Autodesk Inventor part; units mm, degrees
ref_plane "YZ Plane" through (0, 0, 0) normal (1, 0, 0) x (0, 1, 0)
ref_plane "XZ Plane" through (0, 0, 0) normal (0, 1, 0) x (-1, 0, 0)
ref_plane "XY Plane" through (0, 0, 0) normal (0, 0, 1) x (1, 0, 0)
sketch "Esboço1" plane through (0, 0, 0) normal (0, 0, 1) x (1, 0, 0)
  circle A0 centre (0, 0) radius 4
  circle A1 centre (-7, 44.6) radius 3
  circle A2 centre (45, 0) radius 3
  circle A3 centre (-6, -44.6) radius 3
  circle A4 centre (-43.5, 11.3) radius 3
  circle A5 centre (0, 0) radius 29.3573
  circle A6 centre (-7, 44.6) radius 5
  circle A7 centre (-43.5, 11.3) radius 5
  circle A8 centre (-6, -44.6) radius 5
  circle A9 centre (45, 0) radius 5
  line L0 (-12, 44.6) -> (-12, 26.7927)
  line L1 (40.0933, -0.9613) -> (42.8631, -4.0842)
  line L2 (-2.5586, 46.8966) -> (6.9412, 28.5249)
  line L3 (-45.4208, 6.6836) -> (-29.3573, 0)
  line L4 (-42.4056, 16.1788) -> (-26.5097, 12.6129)
  line L5 (-9, -27.9437) -> (-10.963, -43.993)
  line L6 (1.5707, -29.3152) -> (-1.4137, -47.5322)
  line L7 (14.7039, 28.5249) -> (31.099, 28.5249)
  line L8 (31.099, 28.5249) -> (53.6238, -3.5874)
  line L9 (-48.496, 11.5007) -> (-48.496, 11.0993)
  line L10 (14.6238, -44.6) -> (14.6238, -108.4)
  line L11 (53.6238, -44.6) -> (53.6238, -108.4)
  line L12 (53.6238, -108.4) -> (14.6238, -108.4)
  line L13 (65.104, -44.6) -> (65.104, -19.9542)
  line L14 (65.104, -19.9542) -> (49.0934, 2.8713)
  line L15 (14.6238, -44.6) -> (14.6238, -25.4557)
  line L16 (-6, -44.6) -> (-0.9333, -44.6)
  line L17 (14.6238, -44.6) -> (65.104, -44.6)
  line L18 (14.7039, 28.5249) -> (6.9412, 28.5249)
  point P0 (-1, -44.6)
  dimension "d15" = 10
  dimension "d0" = 8
  dimension "d1" = 44.6
  dimension "d2" = 7
  dimension "d3" = 6
  dimension "d4" = 6
  dimension "d5" = 45
  dimension "d6" = 6
  dimension "d7" = 44.6
  dimension "d8" = 6
  dimension "d9" = 11.3
  dimension "d10" = 6
  dimension "d11" = 37.5
  dimension "d12" = 44.6
  dimension "d13" = 10
  dimension "d14" = 10
  dimension "d16" = 10
  dimension "d17" = 0
extrude "Extrusão1" add sketch "Esboço1" along normal blind 20 contours A0
extrude "Extrusão2" add sketch "Esboço1" along normal blind 5 contours A8 | A8 L5 A5 L6 L16 | A5 | L3 A7 L4 A5 | A7 L9 | L0 A6 L2 A5 | A6 picked at (-39.2458, 10.6554)
extrude "Extrusão3" add sketch "Esboço1" along normal mid plane 15 contours A9 | A5 L18 L7 L8 L14 L13 L17 L15 | L17 L11 L12 L10
properties part number "Motor"
Design review of the part built by this model. Coordinates are the model's own, in mm. A direction names the side the tool comes from. Give positions to 0.01 mm unless a question says otherwise; leave off trailing zeros. Write each loop counter-clockwise with the first axis right and the second up, starting at its lowest first coordinate (ties: lowest second). Pieces come first, ordered by that corner, then holes. Notation, with made-up numbers: M 24.25,-36.75 L 78.25,-36.75 A24 cw 78.25,-13.75 Z; hole C 12.25,64 d7. An arc over 180 degrees is marked long. Return JSON: item names as keys, results as strings. Group by question number.
Item 1: Tool access review of faces 4 (the flat face through (53.624, -76, 0)), 5 (the flat face through (-12, 36, 2)), 6 (the cylindrical face through (-0.867, 3.905, 12.395)), 7 (the flat face through (0.336, -36.851, 2.465)), 8 (the cylindrical face through (28.99, 4.62, -3.8)): name each direction out of +Z, -Z, +X, -X, +Y, -Y from which nothing blocks a thin tool from reaching the whole face with its end or side.
Item 2: Clearance check with flat-ended pins moving along their axes: pin 1 Ø5 at (x, y) = (-7, 44.6) entering from -Z; pin 2 Ø1 at (x, z) = (2.5, 1.5) entering from +Y; pin 3 Ø4 at (x, z) = (16, -4) entering from +Y; pin 4 Ø7 at (x, y) = (45, 0) entering from +Z. State where each tip first meets the part, or that it passes through.
Item 3: Take a section at A-A (z = -2.25). Give the boundary of the cut face in (x, y).
Item 4: Take a section at B-B (x = -6). Give the boundary of the cut face in (y, z).
Item 5: Take a section at C-C (y = -61). Give the boundary of the cut face in (x, z), plus the area to 3 significant figures.
Item 6: The part is to be moulded in two halves that separate along X. For faces 1 (the flat face through (59, -44.6, 0)), 2 (the cylindrical face through (-20.622, 20.894, 2.465)), 3 (the cylindrical face through (-8.272, 49.435, 2.465)), say which applies: pulls with the +X half, pulls with the -X half, needs draft (parallel to the pull), parting line crosses it, or undercut.
Item 7: Wall thickness on line 1 along Y through (x, z) = (-6, 2.7); line 2 along Y through (x, z) = (30.5, 0.5); line 3 along Z through (x, y) = (41.5, -98): over which ranges is each line inside the solid? List them lowest first.
Item 8: Take a section at D-D (z = 18). Give the boundary of the cut face in (x, y), plus the area to 3 significant figures.
Return value:
{
 "1": {"face 4": "+Z, -Z, +X, -Y", "face 5": "+Z, -Z, -X, +Y", "face 6": "+Z", "face 7": "+Z, -Z, -Y", "face 8": "-Z, -X"},
 "2": {"pin 1": "passes through", "pin 2": "stops at y = 38.08", "pin 3": "stops at y = 28.52", "pin 4": "stops at z = 7.5"},
 "3": {"outline": "M 6.94,28.52 A29.36 cw 14.62,-25.46 L 14.62,-108.4 L 53.62,-108.4 L 53.62,-44.6 L 65.1,-44.6 L 65.1,-19.95 L 53.62,-3.59 L 31.1,28.52 Z; hole C 45,0 d6"},
 "4": {"outline": "M -49.6,0 L -47.6,0 L -47.6,5 L -49.6,5 Z; M -41.6,0 L 41.77,0 L 41.77,5 L -41.6,5 Z; M 47.43,0 L 49.5,0 L 49.5,5 L 47.43,5 Z"},
 "5": {"outline": "M 14.62,-7.5 L 53.62,-7.5 L 53.62,7.5 L 14.62,7.5 Z", "area": "585 mm2"},
 "6": {"face 1": "needs draft", "face 2": "undercut", "face 3": "parting line crosses it"},
 "7": {"line 1": "y = -49.6 to -47.6, -41.6 to 41.77, 47.43 to 49.5", "line 2": "y = -108.4 to 28.52", "line 3": "z = -7.5 to 7.5"},
 "8": {"outline": "C 0,0 d8", "area": "50.3 mm2"}
}
